```python
from build123d import *

# Parameters (mm, degrees)
F1_DEPTH = 13
F0_R     = 9
F2_DEPTH = 1


with BuildPart() as f1:
    # F0 (on Top) → F1 (new body)
    with BuildSketch(Plane.XY):
        with BuildLine():
            Line((0, 8), (0, -8))
            ThreePointArc((0, -8), (8, 0), (0, 8))
        make_face()
        with BuildLine():
            ThreePointArc((1, 6.928203), (7, 0), (1, -6.928203))
            Line((1, -6.928203), (1, 6.928203))
        make_face(mode=Mode.SUBTRACT)
    extrude(amount=F1_DEPTH)

    # F0 (on Top) → F2 (join)
    with BuildSketch(Plane.XY):
        Circle(F0_R)
        with BuildLine():
            ThreePointArc((0, 8), (8, 0), (0, -8))
            Line((0, -8), (0, 8))
        make_face(mode=Mode.SUBTRACT)
    extrude(amount=F2_DEPTH)


solid = f1.part
```
Here's how the part is built. I have some questions about the finished solid (model axes, mm). A direction names the side the tool comes from. Give positions to 0.01 mm unless a question says otherwise; leave off trailing zeros. Write each loop counter-clockwise with the first axis right and the second up, starting at its lowest first coordinate (ties: lowest second). Pieces come first, ordered by that corner, then holes. Notation, with made-up numbers: (-21, 72.5) -> (10, 72.5) arc R20 ccw to (10, 102.5) -> close; hole circle Ø11 at (33, -16.75). An arc over 180 degrees is marked (long way). Write each question's results on one line, items separated by ' | '.
Item 1: On a 3-axis mill with a long thin cutter (end or side, diameter ignored), from which of +Z, -Z, +X, -X, +Y, -Y can I reach the whole of each face in a straight line? I mean faces 4 (the face through (-1.172, 8.923, 0.493)), 5 (the face through (0, 0, 7)). Say none if no direction works.
Output:
face 4: +Z, -Z | face 5: +Z, -X, +Y, -Y
Item 2: We'd pull the mould along Y, two halves only. Please class faces 1 (the face through (1, 0, 6)), 2 (the face through (8, 0, 7)), 3 (the face through (-2, 0, 1)): pulls with the +Y half, pulls with the -Y half, needs draft (parallel to the pull), parting line crosses it, or undercut.
Output:
face 1: undercut | face 2: parting line crosses it | face 3: needs draft
Item 3: Suppose I cut it at C-C on z = 5. Write out the boundary of the cut face in (x, y).
Output:
outline: (0, -8) arc R8 ccw to (0, 8) -> close; hole (1, -6.93) arc R7 ccw to (1, 6.93) -> close
Item 4: For pin 1 Ø1 at (y, z) = (-4, 9) entering from -X; pin 2 Ø4 at (x, z) = (-6.5, 3.5) entering from +Y; pin 3 Ø4 at (x, y) = (-5.5, 1) entering from +Z, each with a flat end and sliding along its axis, tell me the tip position at first contact or that it passes through.
Output:
pin 1: stops at x = 0 | pin 2: passes through | pin 3: stops at z = 1
Item 5: Suppose I cut it at D-D on x = -4.75. Write out the boundary of the cut face in (y, z), plus the area to 3 significant figures.
Output:
outline: (-7.64, 0) -> (7.64, 0) -> (7.64, 1) -> (-7.64, 1) -> close | area: 15.3 mm^2
Item 6: If I drill on L1, parallel to Z at x = -4.75, y = -7; L2, parallel to Y at x = 2, z = 1.25; L3, parallel to X at y = -2.5, z = 12.5, over which ranges is the centre line in solid material (lowest first)?
Output:
L1: z = 0 to 1 | L2: y = -7.75 to -6.71, 6.71 to 7.75 | L3: x = 0 to 1, 6.54 to 7.6
Item 7: Suppose I cut it at B-B on x = 2.5. Write out the boundary of the cut face in (y, z), plus the area to 3 significant figures.
Output:
outline: (-8.65, 0) -> (-6.54, 0) -> (-6.54, 13) -> (-7.6, 13) -> (-7.6, 1) -> (-8.65, 1) -> close; (6.54, 0) -> (8.65, 0) -> (8.65, 1) -> (7.6, 1) -> (7.6, 13) -> (6.54, 13) -> close | area: 29.7 mm^2
Item 8: Suppose I cut it at A-A on y = 0. Write out the boundary of the cut face in (x, z), plus the area to 3 significant figures.
Output:
outline: (-9, 0) -> (1, 0) -> (1, 13) -> (0, 13) -> (0, 1) -> (-9, 1) -> close; (7, 0) -> (9, 0) -> (9, 1) -> (8, 1) -> (8, 13) -> (7, 13) -> close | area: 36.0 mm^2
